Could you check a few things on this model? Use its own coordinates, in mm. A direction names the side the tool comes from. Round coordinates to 2 decimals unless told otherwise and drop trailing zeros. Loops run counter-clockwise (first coordinate to the right, second up) from the corner with the lowest first, then second, coordinate; pieces in that order, holes last. Notation, with made-up numbers: (32, -11) - (61, -11) arc R11 ccw to (61, 6) - close; hole circle Ø10 at (64.5, 46.25). An arc over 180 degrees is marked (long way). Use one line per item in the form item = value.
```python
from build123d import *

# Parameters (mm, degrees)
BOSS_EXTRUDE1_DEPTH         = 22.225
FILLET1_R                   = 12.7
F_5_8_18_TAPPED_HOLE1_D     = 14.68374
F_5_8_18_TAPPED_HOLE1_DEPTH = 25.4
F_5_8_18_TAPPED_HOLE2_D     = 14.68374
F_5_8_18_TAPPED_HOLE2_DEPTH = 25.4
SKETCH8_W                   = 31.75
SKETCH8_H                   = 25.4
CUT_EXTRUDE1_DEPTH          = 11.43
FILLET2_R                   = 3.429
FILLET2_OF_MIRROR1_R        = 3.429


with BuildPart() as part:
    # Sketch1 → Boss-Extrude1 (new, symmetric)
    with BuildSketch(Plane.XY):
        Polygon((76.2, 0), (0, 0), (0, 25.4), (76.2, 25.4), (76.2, 50.8), (-25.4, 50.8), (-25.4, -38.1), (50.8, -38.1), (50.8, -63.5), (-25.4, -63.5), (-25.4, -88.9), (76.2, -88.9), align=None)
    extrude(amount=BOSS_EXTRUDE1_DEPTH, both=True)

    # Fillet1
    fillet1_edges = [part.edges().sort_by_distance(p)[0] for p in [
        (50.8, -63.5, 0),
        (50.8, -38.1, 0),
        (0, 25.4, 0),
        (0, 0, 0),
    ]]
    fillet(fillet1_edges, radius=FILLET1_R - 0.0001)  # a hair under: the kernel refuses the full size

    # 5/8-18 Tapped Hole1
    with Locations(Plane.XZ.offset(88.9)):
        with Locations((25.4, 0)):
            Hole(F_5_8_18_TAPPED_HOLE1_D / 2, depth=F_5_8_18_TAPPED_HOLE1_DEPTH)

    # 5/8-18 Tapped Hole2
    with Locations(Plane(origin=(0, 50.8, 0), x_dir=(-1, 0, 0), z_dir=(0, 1, 0))):
        with Locations((-25.4, 0)):
            Hole(F_5_8_18_TAPPED_HOLE2_D / 2, depth=F_5_8_18_TAPPED_HOLE2_DEPTH)

    # Sketch8 → Cut-Extrude1 (cut)
    with BuildSketch(Plane.XY.offset(22.225)):
        with Locations((25.4, -19.05)):
            Rectangle(SKETCH8_W, SKETCH8_H)
    cut_extrude1 = extrude(amount=-CUT_EXTRUDE1_DEPTH, mode=Mode.SUBTRACT)

    # Fillet2
    fillet2_edges = [part.edges().sort_by_distance(p)[0] for p in [
        (41.275, -6.35, 16.51),
        (41.275, -31.75, 16.51),
        (9.525, -31.75, 16.51),
        (9.525, -6.35, 16.51),
    ]]
    fillet(fillet2_edges, radius=FILLET2_R)

    # Mirror1: Cut-Extrude1 across plane
    add(cut_extrude1.mirror(Plane.XY), mode=Mode.SUBTRACT)

    # Fillet2 of Mirror1
    fillet2_of_mirror1_edges = [part.edges().sort_by_distance(p)[0] for p in [
        (41.275, -6.35, -16.51),
        (41.275, -31.75, -16.51),
        (9.525, -31.75, -16.51),
        (9.525, -6.35, -16.51),
    ]]
    fillet(fillet2_of_mirror1_edges, radius=FILLET2_OF_MIRROR1_R)


solid = part.part
```
1. If we section it at A-A, the plane x = 63: Write out the boundary of the cut face in (y, z) (3 decimals), plus the area to 3 significant figures.
Solution:
outline = (-88.9, -22.225) - (0, -22.225) - (0, 22.225) - (-88.9, 22.225) - close; (25.4, -22.225) - (50.8, -22.225) - (50.8, 22.225) - (25.4, 22.225) - close
area = 5,080 mm^2
2. Please list where these lines run through material, in increasing order: line 1 along Y through (x, z) = (35, 12.5); line 2 along Y through (x, z) = (38.5, -1); line 3 along Y through (x, z) = (55, -15).
Solution:
line_1 = -88.9 to -63.5, -38.1 to -31.75, -6.35 to 0, 25.4 to 50.8
line_2 = -88.9 to -63.49, -38.11 to 0, 25.4 to 50.8
line_3 = -88.9 to 0, 25.4 to 50.8
3. If we section it at C-C, the plane x = 23: Write out the boundary of the cut face in (y, z) (3 decimals).
Solution:
outline = (-88.9, -22.225) - (-63.5, -22.225) - (-63.5, -6.939) - (-88.9, -6.939) - close; (-88.9, 6.939) - (-63.5, 6.939) - (-63.5, 22.225) - (-88.9, 22.225) - close; (-38.1, -22.225) - (-31.75, -22.225) - (-31.75, -10.795) - (-6.35, -10.795) - (-6.35, -22.225) - (0, -22.225) - (0, 22.225) - (-6.35, 22.225) - (-6.35, 10.795) - (-31.75, 10.795) - (-31.75, 22.225) - (-38.1, 22.225) - close; (25.4, -22.225) - (50.8, -22.225) - (50.8, -6.939) - (25.4, -6.939) - close; (25.4, 6.939) - (50.8, 6.939) - (50.8, 22.225) - (25.4, 22.225) - close
4. For P1, Ø12.5, axis at x = 20.5, y = -13.5, coming from the -Z side (3 decimals); P2, Ø23.5, axis at x = 25.4, z = 0, coming from the -Y side, each with a flat end and sliding along its axis, tell me the tip position at first contact or that it passes through.
Solution:
P1 = -10.795
P2 = -88.9
5. On a 3-axis mill with a long thin cutter (end or side, diameter ignored), from which of +Z, -Z, +X, -X, +Y, -Y can I reach the whole of each face in a straight line? I mean faces 1 (the face through (76.2, 38, 0)), 2 (the face through (10.556, -30.772, 16.43)), 3 (the face through (47.18, -41.92, 0.31)), 4 (the face through (3.82, 3.62, 0.31)), 5 (the face through (10.556, -7.328, -16.43)). Say none if no direction works.
Solution:
face_1 = +Z, -Z, +X, +Y, -Y
face_2 = +Z
face_3 = +Z, -Z, -X
face_4 = +Z, -Z, +X
face_5 = -Z
6. We'd pull the mould along Z, two halves only. Please class faces 6 (the face through (10.556, -30.772, -16.43)), 7 (the face through (22.012, -76.022, -6.514)), 8 (the face through (18.065, 37.922, 0.323)), 9 (the face through (25, -19, -10.795)): +Z half, -Z half, draft (parallel to the pull), parting line (faces both ways), or undercut.
Solution:
face_6 = draft
face_7 = undercut
face_8 = undercut
face_9 = -Z half
7. If we section it at B-B, the plane z = 0: Count the separate pieces of the cut face and the enclosed holes in it, plus the area to 3 significant figures.
Solution:
separate_pieces = 3
enclosed_holes = 0
area = 9,720 mm^2
